Autodesk Inventor part; units mm, degrees
ref_plane "YZ Plane" through (0, 0, 0) normal (1, 0, 0) x (0, 1, 0)
ref_plane "XZ Plane" through (0, 0, 0) normal (0, 1, 0) x (-1, 0, 0)
ref_plane "XY Plane" through (0, 0, 0) normal (0, 0, 1) x (1, 0, 0)
sketch "Esboço1" plane through (0, 0, 0) normal (0, 0, 1) x (1, 0, 0)
  line L0 (27.5, -14.5) -> (-27.5, -14.5)
  line L1 (-27.5, -14.5) -> (-27.5, 14.5)
  line L2 (-27.5, 14.5) -> (27.5, 14.5)
  line L3 (27.5, 14.5) -> (27.5, -14.5)
  line L4 (27.5, -14.5) -> (-27.5, 14.5) construction
  line L5 (-27.5, -14.5) -> (27.5, 14.5) construction
  point P0 (0, 0)
  dimension "d0" = 55
  dimension "d1" = 29
extrude "Extrusão1" add sketch "Esboço1" along normal blind 5
sketch "Esboço2" plane through (0, 0, 5) normal (0, 0, 1) x (1, 0, 0)
  line L0 (-27.5, 14.5) -> (-27.5, -14.5)
  line L1 (27.5, 14.5) -> (-27.5, 14.5)
  line L2 (0, 0) -> (-7.3879, 0)
  line L3 (0, 0) -> (0, 5.1516)
  point P0 (-17.5, 10.25)
  point P1 (17.5, 10.25)
  point P2 (-17.5, -10.25)
  point P3 (17.5, -10.25)
  dimension "d4" = 10
  dimension "d5" = 4.25
hole "Furo1" at (-17.5, 10.25, 5) at (17.5, 10.25, 5) at (-17.5, -10.25, 5) at (17.5, -10.25, 5) direction (0, 0, -1) diameter 4 end through all countersink diameter 6 countersink angle 90
properties part number "Tampa Apoio Motor" material "Plástico PC/ABS"
Part model, mm, in its own coordinate system. Coordinates: 2 decimals unless noted, no trailing zeros. Write each loop counter-clockwise with the first axis right and the second up, starting at its lowest first coordinate (ties: lowest second). Pieces come first, ordered by that corner, then holes.
Item 1: Probe line 1 (Y direction, x = -17.5, z = 2.55); line 2 (X direction, y = 10.25, z = 0.8); line 3 (X direction, y = 8.25, z = 4.65). List the from-to ranges inside material, lowest first.
Item 2: Slice it at A-A (z = 0.65). Write the cut outline in (x, y).
Item 3: Slice it at C-C (x = 17.5). Write the cut outline in (y, z), and give its area (3 significant figures).
Item 4: Slice it at B-B (y = -10.25). Write the cut outline in (x, z).
Item 5: Pin check, flat tip, straight feed: pin 1 (5 mm diameter, centred on x = -17.5, y = 10.25, fed in from +Z). Stop position of the tip, or through.
Item 6: Mould opens along Y. For faces 1 (the face through (0, 0, 0)), 2 (the face through (-19.483, 10.51, 1.972)), 3 (the face through (0, -14.5, 2)) say: released by +Y, released by -Y, zero draft, split by the parting line, or undercut.
Results found:
1. line 1: y = -14.5 to -12.25, -8.25 to 8.25, 12.25 to 14.5
1. line 2: x = -27.5 to -19.5, -15.5 to 15.5, 19.5 to 27.5
1. line 3: x = -27.5 to -19.24, -15.76 to 15.76, 19.24 to 27.5
2. outline: (-27.5, -14.5) - (27.5, -14.5) - (27.5, 14.5) - (-27.5, 14.5) - close; hole circle Ø4 at (-17.5, -10.25); hole circle Ø4 at (-17.5, 10.25); hole circle Ø4 at (17.5, -10.25); hole circle Ø4 at (17.5, 10.25)
3. outline: (-14.5, 0) - (-12.25, 0) - (-12.25, 4) - (-13.25, 5) - (-14.5, 5) - close; (-8.25, 0) - (8.25, 0) - (8.25, 4) - (7.25, 5) - (-7.25, 5) - (-8.25, 4) - close; (12.25, 0) - (14.5, 0) - (14.5, 5) - (13.25, 5) - (12.25, 4) - close
3. area: 103 mm2
4. outline: (-27.5, 0) - (-19.5, 0) - (-19.5, 4) - (-20.5, 5) - (-27.5, 5) - close; (-15.5, 0) - (15.5, 0) - (15.5, 4) - (14.5, 5) - (-14.5, 5) - (-15.5, 4) - close; (19.5, 0) - (27.5, 0) - (27.5, 5) - (20.5, 5) - (19.5, 4) - close
5. pin 1: stops at z = 4.5
6. face 1: zero draft
6. face 2: undercut
6. face 3: released by -Y
